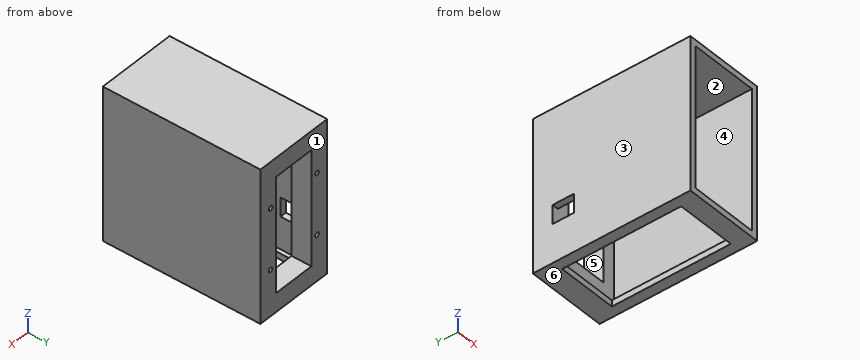
Autodesk Inventor part; units mm, degrees
ref_plane "YZ Plane" through (0, 0, 0) normal (1, 0, 0) x (0, 1, 0)
ref_plane "XZ Plane" through (0, 0, 0) normal (0, 1, 0) x (-1, 0, 0)
ref_plane "XY Plane" through (0, 0, 0) normal (0, 0, 1) x (1, 0, 0)
sketch "Sketch1" plane through (0, 0, 0) normal (0, 1, 0) x (-1, 0, 0)
  line L0 (0, 0) -> (-250, 0)
  line L1 (-250, 0) -> (-250, -520)
  line L2 (-250, -520) -> (0, -520)
  line L3 (0, -520) -> (0, 0)
  line L4 (23, -543) -> (-273, -543)
  line L5 (-273, -543) -> (-273, 23)
  line L6 (-273, 23) -> (23, 23)
  line L7 (23, 23) -> (23, -543)
  dimension "d0" = 250
  dimension "d1" = 520
  dimension "d2" = 23
extrude "Extrusion1" add sketch "Sketch1" along normal blind 583
sketch "Sketch2" plane through (273, 0, -543) normal (0, 0, -1) x (-1, 0, 0)
  line L0 (38, 506) -> (258, 506)
  line L1 (258, 506) -> (258, 66)
  line L2 (258, 66) -> (38, 66)
  line L3 (38, 66) -> (38, 506)
  line L4 (0, 583) -> (296, 583)
  line L5 (296, 0) -> (296, 583)
  point P0 (273, 0)
  dimension "d5" = 220
  dimension "d6" = 440
  dimension "d7" = 77
  dimension "d8" = 38
extrude "Extrusion2" cut sketch "Sketch2" against normal up to surface (23 mm away)
sketch "Sketch3" plane through (-23, 0, -543) normal (-1, 0, 0) x (0, 0, 1)
  line L0 (143, 510) -> (213, 510)
  line L1 (213, 510) -> (213, 430)
  line L2 (213, 430) -> (143, 430)
  line L3 (143, 430) -> (143, 510)
  line L4 (566, 0) -> (0, 0)
  line L5 (0, 0) -> (0, 583)
  point P0 (543, 0)
  dimension "d11" = 70
  dimension "d12" = 80
  dimension "d13" = 430
  dimension "d14" = 143
extrude "Extrusion3" cut sketch "Sketch3" against normal up to surface (23 mm away)
sketch "Sketch5" plane through (0, 583, 0) normal (0, 1, 0) x (1, 0, 0)
  line L0 (250, 0) -> (250, 520)
  line L1 (250, 520) -> (0, 520)
  line L2 (250, 0) -> (0, 0)
  line L3 (0, 0) -> (0, 520)
  line L4 (0, 520) -> (250, 520)
  line L5 (250, 520) -> (250, 0)
  line L6 (47, 47) -> (203, 47)
  line L7 (203, 47) -> (203, 473)
  line L8 (203, 473) -> (47, 473)
  line L9 (47, 473) -> (47, 47)
  dimension "d17" = 47
extrude "Extrusion4" add sketch "Sketch5" against normal up to surface (73 mm away)
sketch "Sketch6" plane through (0, 583, 0) normal (0, 1, 0) x (1, 0, 0)
  circle A0 centre (228, 373) radius 8
  line L0 (273, 543) -> (-23, 543)
  line L1 (273, -23) -> (273, 543)
  circle A1 centre (228, 147) radius 8
  line L2 (-23, -23) -> (273, -23)
  line L3 (125, -23) -> (125, 543) construction
  circle A2 centre (22, 373) radius 8
  circle A3 centre (22, 147) radius 8
  point P0 (0, 0)
  dimension "d20" = 16
  dimension "d21" = 170
  dimension "d22" = 45
  dimension "d23" = 16
  dimension "d24" = 170
  dimension "d25" = 45
extrude "Extrusion5" cut sketch "Sketch6" against normal blind 10
properties part number "Riight Leg" material "Iron, Cast"
Geometry check sheet. Reference: the model listing, model coordinates, mm. Face numbers are marked on the shaded views. A direction names the side the tool comes from. Coordinates: 2 decimals unless noted, no trailing zeros. Order: outer loops, then holes, each group sorted by start corner. A loop starts at its lowest first (then second) coordinate and runs counter-clockwise, first axis right, second up.
Q1. Sectioned sample at C-C on x = 137.5. Record the cut outline in (y, z).
Reply:
outline: (0, -543) - (66, -543) - (66, -520) - (0, -520) - close; (0, 0) - (510, 0) - (510, -47) - (583, -47) - (583, 23) - (0, 23) - close; (506, -543) - (583, -543) - (583, -473) - (510, -473) - (510, -520) - (506, -520) - close
Q2. Sectioned sample at A-A on z = -147. Record the cut outline in (x, y).
Reply:
outline: (-23, 0) - (0, 0) - (0, 510) - (47, 510) - (47, 583) - (30, 583) - (30, 573) - (14, 573) - (14, 583) - (-23, 583) - close; (203, 510) - (250, 510) - (250, 0) - (273, 0) - (273, 583) - (236, 583) - (236, 573) - (220, 573) - (220, 583) - (203, 583) - close
Q3. Tool access check on the marked faces 4, 5 and 6. Record the directions out of +Z, -Z, +X, -X, +Y, -Y that give a thin tool (end or side, any length) a straight path to the whole face; none if there is none.
Reply:
face 4: -Y
face 5: +Y, -Y
face 6: -Z, +X, -X, +Y, -Y
Q4. Depth check by flat-ended pin: pin 1 Ø17.5 at (x, z) = (23.5, -146) entering from +Y; pin 2 Ø9.5 at (x, z) = (22, -373) entering from -Y; pin 3 Ø5 at (x, z) = (225, -373.5) entering from +Y; pin 4 Ø1 at (x, z) = (178.5, -472) entering from -Y. Enter the tip coordinate at first touch or a pass-through.
Reply:
pin 1: stops at y = 583
pin 2: stops at y = 510
pin 3: stops at y = 573
pin 4: passes through
Q5. Thickness scan on probe 1 along X at (y, z) = (576, -147); probe 2 along Z at (x, y) = (22, 579); probe 3 along X at (y, z) = (210, -511.5). Record the ranges inside material, lowest first.
Reply:
probe 1: x = -23 to 14, 30 to 47, 203 to 220, 236 to 273
probe 2: z = -543 to -381, -365 to -155, -139 to 23
probe 3: x = -23 to 0, 250 to 273
Q6. Sectioned sample at D-D on z = -373. Record the cut outline in (x, y), and give its area (3 significant figures).
Reply:
outline: (-23, 0) - (0, 0) - (0, 430) - (-23, 430) - close; (-23, 510) - (47, 510) - (47, 583) - (30, 583) - (30, 573) - (14, 573) - (14, 583) - (-23, 583) - close; (203, 510) - (250, 510) - (250, 0) - (273, 0) - (273, 583) - (236, 583) - (236, 573) - (220, 573) - (220, 583) - (203, 583) - close
area: 31,500 mm2
Q7. Draft check along X on the marked faces 1, 2 and 3. Enter one of: released by +X, released by -X, zero draft, split by the parting line, or undercut.
Reply:
face 1: zero draft
face 2: undercut
face 3: released by -X
Q8. Sectioned sample at B-B on x = 228. Record the cut outline in (y, z).
Reply:
outline: (0, -543) - (66, -543) - (66, -520) - (0, -520) - close; (0, 0) - (510, 0) - (510, -520) - (506, -520) - (506, -543) - (583, -543) - (583, -381) - (573, -381) - (573, -365) - (583, -365) - (583, -155) - (573, -155) - (573, -139) - (583, -139) - (583, 23) - (0, 23) - close
